Geometry check sheet. Reference: the model listing, model coordinates, mm. A direction names the side the tool comes from. Coordinates: 2 decimals unless noted, no trailing zeros. Write each loop counter-clockwise with the first axis right and the second up, starting at its lowest first coordinate (ties: lowest second). Pieces come first, ordered by that corner, then holes. Notation, with made-up numbers: M 22,77.25 L 65,77.25 A26 ccw 65,113.25 Z; hole C 3,-40 d2. An arc over 180 degrees is marked long. Put each result on its own line as item: value. Start each with the question number.
1) Gauge pin test, flat ends, axial feed: pin 1 (0.8 mm diameter, centred on y = 10.5, z = -39, fed in from -X); pin 2 (5.5 mm diameter, centred on y = -5, z = 33.5, fed in from +X). Record the tip position at first contact, or that the pin passes through.
2) Set-up check for faces 4 (the flat face through (-62, -5, 34)), 5 (the flat face through (64, -5, 37)), 6 (the flat face through (-33, 12, 38.5)), 7 (the flat face through (64, -5, -37)), 8 (the flat face through (-67, -5, 34)): record each of +Z, -Z, +X, -X, +Y, -Y from which the full face is reachable in a straight line by a thin tool's end or side.
3) Mould release check, pull along X, two halves, no side actions. Record for faces 1 (the flat face through (-1, 13, -40)), 2 (the flat face through (-70, 13, 1)), 3 (the cylindrical face through (-67.6, 13.66, -37.64)): released by +X, released by -X, zero draft, split by the parting line, or undercut.
4) Cross-section at D-D on z = -2.5. Record the cut outline in (x, y), plus the area to 3 significant figures.
5) Cross-section at C-C on y = 6. Count the separate pieces of the cut face and the enclosed holes in it, plus the area to 3 significant figures.
6) Cross-section at A-A on x = 23.5. Record the cut outline in (y, z), plus the area to 3 significant figures.
7) Scan lines: line 1 along Z through (x, y) = (-58, 5); line 2 along X through (y, z) = (8.5, 4); line 3 along Y through (x, z) = (5.5, 34.5). Record each from-to range of solid material in increasing order.
8) Cross-section at B-B on z = 20. Record the cut outline in (x, y).
from build123d import *

# Parameters (mm, degrees)
SKETCH1_W           = 140
SKETCH1_H           = 80
BOSS_EXTRUDE1_DEPTH = 2
SKETCH2_W           = 45.094685242
SKETCH2_H           = 1.5
SKETCH2_W_2         = 45.594685242
BOSS_EXTRUDE3_DEPTH = 23
SKETCH3_W           = 140
SKETCH3_H           = 80
BOSS_EXTRUDE4_DEPTH = 1.5
SKETCH4_R           = 3.5
CUT_EXTRUDE1_DEPTH  = 5
FILLET1_R           = 3
SKETCH5_W           = 5
SKETCH5_H           = 5
BOSS_EXTRUDE5_DEPTH = 10


with BuildPart() as part:
    # Sketch1 → Boss-Extrude1 (new body)
    with BuildSketch(Plane(origin=(0, 0, 0), x_dir=(1, 0, 0), z_dir=(0, 1, 0))):
        Rectangle(SKETCH1_W, SKETCH1_H)
        Polygon((68.5, -18), (68.5, 17), (30, 17), (30, 38.5), (-58.5, 38.5), (-58.5, 28.5), (-68.5, 28.5), (-68.5, -28.5), (-58.5, -28.5), (-58.5, -38.5), (-40, -38.5), (-40, -18), align=None, mode=Mode.SUBTRACT)
    extrude(amount=BOSS_EXTRUDE1_DEPTH)

    # Sketch2 → Boss-Extrude3 (add)
    with BuildSketch(Plane(origin=(0, 2, 0), x_dir=(1, 0, 0), z_dir=(0, 1, 0))):
        with Locations((-23.047342621, 39.25)):
            Rectangle(SKETCH2_W, SKETCH2_H)
        with Locations((-23.047342621, -39.25)):
            Rectangle(SKETCH2_W, SKETCH2_H)
        Polygon((-46.094685242, 40), (-46.094685242, 38.5), (-68.5, 38.5), (-68.5, -38.5), (-46.094685242, -38.5), (-46.094685242, -40), (-70, -40), (-70, 40), align=None)
        with Locations((22.797342621, -39.25)):
            Rectangle(SKETCH2_W_2, SKETCH2_H)
        Polygon((46.094685242, -38.5), (46.094685242, -40), (70, -40), (70, 40), (46.094685242, 40), (46.094685242, 38.5), (68.5, 38.5), (68.5, -38.5), align=None)
        with Locations((22.797342621, 39.25)):
            Rectangle(SKETCH2_W_2, SKETCH2_H)
    extrude(amount=BOSS_EXTRUDE3_DEPTH)

    # Sketch3 → Boss-Extrude4 (add)
    with BuildSketch(Plane(origin=(0, 25, 0), x_dir=(1, 0, 0), z_dir=(0, 1, 0))):
        Rectangle(SKETCH3_W, SKETCH3_H)
    extrude(amount=BOSS_EXTRUDE4_DEPTH)

    # Sketch4 → Cut-Extrude1 (cut)
    with BuildSketch(Plane(origin=(70, 0, 0), x_dir=(0, 0, -1), z_dir=(1, 0, 0))):
        with Locations((31, 6)):
            Circle(SKETCH4_R)
    extrude(amount=-CUT_EXTRUDE1_DEPTH, mode=Mode.SUBTRACT)

    # Fillet1
    fillet1_edges = [part.edges().sort_by_distance(p)[0] for p in [
        (70, 13.25, 40),
        (-70, 13.25, 40),
        (-70, 13.25, -40),
        (70, 13.25, -40),
        (-68.5, 13.5, 38.5),
        (-68.5, 13.5, -38.5),
    ]]
    fillet(fillet1_edges, radius=FILLET1_R)

    # Sketch5 → Boss-Extrude5 (add)
    with BuildSketch(Plane.XZ):
        with Locations((-64.5, 34.5)):
            Rectangle(SKETCH5_W, SKETCH5_H)
        with Locations((64.5, 34.5)):
            Rectangle(SKETCH5_W, SKETCH5_H)
        with Locations((64.5, -34.5)):
            Rectangle(SKETCH5_W, SKETCH5_H)
        with Locations((-64.5, -34.5)):
            Rectangle(SKETCH5_W, SKETCH5_H)
    extrude(amount=BOSS_EXTRUDE5_DEPTH)


solid = part.part
Answer key:
1. pin 1: stops at x = -69.54
1. pin 2: stops at x = 67
2. face 4: +Z, -Z, -Y
2. face 5: +Z, +X, -X, -Y
2. face 6: none
2. face 7: -Z, +X, -X, -Y
2. face 8: +Z, -Z, -X, -Y
3. face 1: zero draft
3. face 2: released by -X
3. face 3: undercut
4. outline: M -70,0 L -68.5,0 L -68.5,25 L 68.5,25 L 68.5,0 L 70,0 L 70,26.5 L -70,26.5 Z
4. area: 285 mm²
5. separate pieces: 7
5. enclosed holes: 0
5. area: 632 mm²
6. outline: M 0,-40 L 26.5,-40 L 26.5,40 L 0,40 L 0,18 L 2,18 L 2,38.5 L 25,38.5 L 25,-38.5 L 0,-38.5 Z
6. area: 236 mm²
7. line 1: z = -40 to -38.5, 38.5 to 40
7. line 2: x = -70 to -68.5, 68.5 to 70
7. line 3: y = 0 to 2, 25 to 26.5
8. outline: M -70,0 L -68.5,0 L -68.5,25 L 68.5,25 L 68.5,2 L -40,2 L -40,0 L 70,0 L 70,26.5 L -70,26.5 Z
